Part model, mm, in its own coordinate system. Face numbers are marked on the shaded views. A direction names the side the tool comes from. Coordinates: 2 decimals unless noted, no trailing zeros. Loops run counter-clockwise (first coordinate to the right, second up) from the corner with the lowest first, then second, coordinate; pieces in that order, holes last. Notation, with made-up numbers: (-25, 49.25) - (-3, 49.25) arc R11 ccw to (-3, 67.25) - close; hole circle Ø10 at (15, 18). An arc over 180 degrees is marked (long way). Answer as CSV lines item,"result".
from build123d import *

# Parameters (mm, degrees)
F0_W     = 150
F0_H     = 30
F2_DEPTH = 8
F3_DEPTH = 30


with BuildPart() as f2:
    # F0 (on Top) → F2 (new body)
    with BuildSketch(Plane.XY):
        with Locations((75, 15)):
            Rectangle(F0_W, F0_H)
    extrude(amount=F2_DEPTH)

    # F1 (on Front) → F3 (join)
    with BuildSketch(Plane.XZ):
        Polygon((28, 8), (20, 16), (20, 8), align=None)
        Polygon((56, 8), (48, 16), (48, 8), align=None)
        Polygon((84, 8), (76, 16), (76, 8), align=None)
        Polygon((112, 8), (104, 16), (104, 8), align=None)
        Polygon((140, 8), (132, 16), (132, 8), align=None)
    extrude(amount=-F3_DEPTH)


solid = f2.part
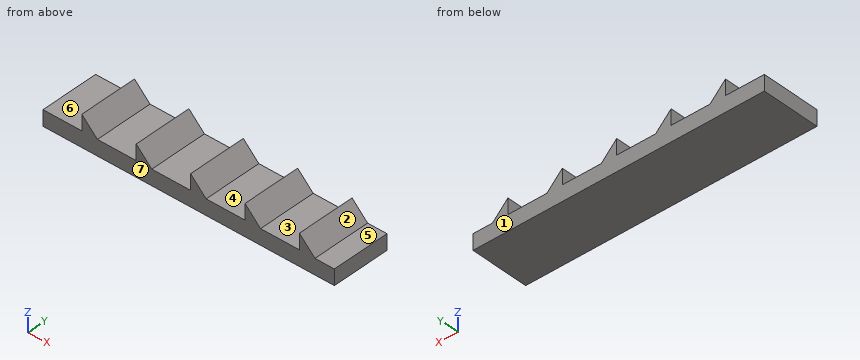
Q1. Saw through at D-D (x = 25.5). Give the cut face in (y, z).
Results:
outline,"(0, 0) - (30, 0) - (30, 10.5) - (0, 10.5) - close"
Q2. Two-plate mould, pull along X, no slides. Class the marked faces 1, 2 and 3: released by +X, released by -X, zero draft, split by the parting line, or undercut.
Results:
face 1,"zero draft"
face 2,"released by +X"
face 3,"undercut"
Q3. Saw through at C-C (x = 78). Give the cut face in (y, z).
Results:
outline,"(0, 0) - (30, 0) - (30, 14) - (0, 14) - close"
Q4. Wall check: L1, parallel to X at y = 15.75, z = 8.5; L2, parallel to X at y = 17.75, z = 14.5; L3, parallel to Z at x = 16, y = 3.25. Give the ranges that are in metal, low to high.
Results:
L1,"x = 20 to 27.5, 48 to 55.5, 76 to 83.5, 104 to 111.5, 132 to 139.5"
L2,"x = 20 to 21.5, 48 to 49.5, 76 to 77.5, 104 to 105.5, 132 to 133.5"
L3,"z = 0 to 8"
Q5. Which spindle directions (+Z, -Z, +X, -X, +Y, -Y) get a long thin tool onto all of the face, cutting with end or side? Do the marked faces 4, 5, 6 and 7. Say none if no direction does.
Results:
face 4,"+Z, +Y, -Y"
face 5,"+Z, +X, +Y, -Y"
face 6,"+Z, -X, +Y, -Y"
face 7,"+Z, -Z, +X, -X, -Y"
Q6. Flat gauge pins, fed straight in: pin 1 (6 mm diameter, centred on y = 21.5, z = 13, fed in from -X); pin 2 (12 mm diameter, centred on x = 63, y = 13.5, fed in from +Z); pin 3 (1.5 mm diameter, centred on y = 14.5, z = 11, fed in from +X). Where does each tip first touch, or does it go through?
Results:
pin 1,"stops at x = 20"
pin 2,"stops at z = 8"
pin 3,"stops at x = 137.75"
Q7. Saw through at A-A (z = 12.25). Give the cut face in (x, y).
Results:
outline,"(20, 0) - (23.75, 0) - (23.75, 30) - (20, 30) - close; (48, 0) - (51.75, 0) - (51.75, 30) - (48, 30) - close; (76, 0) - (79.75, 0) - (79.75, 30) - (76, 30) - close; (104, 0) - (107.75, 0) - (107.75, 30) - (104, 30) - close; (132, 0) - (135.75, 0) - (135.75, 30) - (132, 30) - close"
Q8. Saw through at B-B (y = 17.75). Give the cut face in (x, z).
Results:
outline,"(0, 0) - (150, 0) - (150, 8) - (140, 8) - (132, 16) - (132, 8) - (112, 8) - (104, 16) - (104, 8) - (84, 8) - (76, 16) - (76, 8) - (56, 8) - (48, 16) - (48, 8) - (28, 8) - (20, 16) - (20, 8) - (0, 8) - close"
